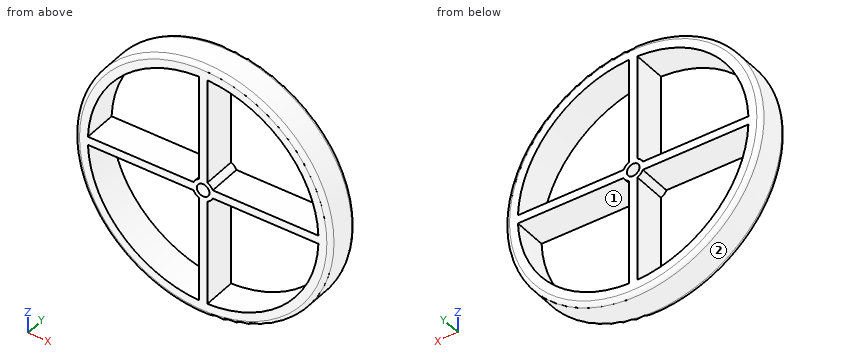
```python
from build123d import *

# Parameters (mm, degrees)
F0_R     = 30.5
F0_R_2   = 1.5000000096
F1_DEPTH = 4
F2_R     = 1


with BuildPart() as f1:
    # F0 (on Front) → F1 (new body, symmetric)
    with BuildSketch(Plane.XZ):
        Circle(F0_R)
        with BuildLine():
            Line((-27.4818121673, -1), (-2.2912878475, -1))
            ThreePointArc((-2.2912878475, -1), (-1.767766953, -1.767766953), (-1, -2.2912878475))
            Line((-1, -2.2912878475), (-1, -27.4818121673))
            ThreePointArc((-1, -27.4818121673), (-19.4454364826, -19.4454364826), (-27.4818121673, -1))
        make_face(mode=Mode.SUBTRACT)
        with BuildLine():
            ThreePointArc((1, -2.2912878475), (1.767766953, -1.767766953), (2.2912878475, -1))
            Line((2.2912878475, -1), (27.4818121673, -1))
            ThreePointArc((27.4818121673, -1), (19.4454364826, -19.4454364826), (1, -27.4818121673))
            Line((1, -27.4818121673), (1, -2.2912878475))
        make_face(mode=Mode.SUBTRACT)
        with BuildLine():
            ThreePointArc((-1, 2.2912878475), (-1.767766953, 1.767766953), (-2.2912878475, 1))
            Line((-2.2912878475, 1), (-27.4818121673, 1))
            ThreePointArc((-27.4818121673, 1), (-19.4454364826, 19.4454364826), (-1, 27.4818121673))
            Line((-1, 27.4818121673), (-1, 2.2912878475))
        make_face(mode=Mode.SUBTRACT)
        Circle(F0_R_2, mode=Mode.SUBTRACT)
        with BuildLine():
            ThreePointArc((1, 27.4818121673), (19.4454364826, 19.4454364826), (27.4818121673, 1))
            Line((27.4818121673, 1), (2.2912878475, 1))
            ThreePointArc((2.2912878475, 1), (1.767766953, 1.767766953), (1, 2.2912878475))
            Line((1, 2.2912878475), (1, 27.4818121673))
        make_face(mode=Mode.SUBTRACT)
    extrude(amount=F1_DEPTH, both=True)

    # F2
    f2_edges = [f1.edges().sort_by_distance(p)[0] for p in [
        (-30.5, -4, 0),
        (-30.5, 4, 0),
    ]]
    fillet(f2_edges, radius=F2_R)


solid = f1.part
```
Here's how the part is built. I have some questions about the finished solid (model axes, mm). Face numbers are marked on the shaded views. Give positions to 0.01 mm unless a question says otherwise; leave off trailing zeros. Write each loop counter-clockwise with the first axis right and the second up, starting at its lowest first coordinate (ties: lowest second). Pieces come first, ordered by that corner, then holes. Notation, with made-up numbers: (59.25, 89) -> (108.25, 89) arc R30 ccw to (108.25, 119) -> close; hole circle Ø11 at (1.25, 4.5). An arc over 180 degrees is marked (long way). Use one line per item in the form item = value.
1) Suppose I cut it at C-C (y = 1.5). Please give me the cut outline in (x, z), and give its area (3 significant figures).
Verdict:
outline = circle Ø61 at (0, 0); hole (-27.48, -1) arc R27.5 ccw to (-1, -27.48) -> (-1, -2.29) arc R2.5 cw to (-2.29, -1) -> close; hole (-27.48, 1) -> (-2.29, 1) arc R2.5 cw to (-1, 2.29) -> (-1, 27.48) arc R27.5 ccw to start; hole circle Ø3 at (0, 0); hole (1, -27.48) arc R27.5 ccw to (27.48, -1) -> (2.29, -1) arc R2.5 cw to (1, -2.29) -> close; hole (1, 2.29) arc R2.5 cw to (2.29, 1) -> (27.48, 1) arc R27.5 ccw to (1, 27.48) -> close
area = 760 mm2
2) Suppose I cut it at A-A (x = 0). Please give me the cut outline in (y, z).
Verdict:
outline = (-4, -29.5) arc R1 ccw to (-3, -30.5) -> (3, -30.5) arc R1 ccw to (4, -29.5) -> (4, -1.5) -> (-4, -1.5) -> close; (-4, 1.5) -> (4, 1.5) -> (4, 29.5) arc R1 ccw to (3, 30.5) -> (-3, 30.5) arc R1 ccw to (-4, 29.5) -> close
3) We'd pull the mould along X, two halves only. Please class the marked faces 1 and 2: +X half, -X half, draft (parallel to the pull), parting line (faces both ways), or undercut.
Verdict:
face_1 = undercut
face_2 = parting line
4) I'm going to push flat-ended pins straight in: pin 1 (1.5 mm diameter, centred on x = -11, y = -2.5, fed in from -Z); pin 2 (2.5 mm diameter, centred on y = -1.5, z = -8.5, fed in from +X); pin 3 (4 mm diameter, centred on y = 1, z = 14.5, fed in from +X). Where does each tip first touch, or does it pass through?
Verdict:
pin_1 = -28.73
pin_2 = 29.63
pin_3 = 27.82
5) If I drill on L1, parallel to Z at x = 0, y = 2.75; L2, parallel to X at y = 3.75, z = -3.5; L3, parallel to Z at x = 17, y = 3, over which ranges is the centre line in solid material (lowest first)? Write a range as [from, to].
Verdict:
L1 = [-30.5, -1.5], [1.5, 30.5]
L2 = [-29.96, -27.28], [-1, 1], [27.28, 29.96]
L3 = [-25.32, -21.62], [-1, 1], [21.62, 25.32]
6) Suppose I cut it at D-D (z = -23). Give the number of separate pieces and of enclosed holes in the cut face, and give its area (3 significant figures).
Verdict:
separate_pieces = 3
enclosed_holes = 0
area = 94.0 mm2
7) Suppose I cut it at B-B (z = 0). Please give me the cut outline in (x, y).
Verdict:
outline = (-30.5, -3) arc R1 ccw to (-29.5, -4) -> (-1.5, -4) -> (-1.5, 4) -> (-29.5, 4) arc R1 ccw to (-30.5, 3) -> close; (1.5, -4) -> (29.5, -4) arc R1 ccw to (30.5, -3) -> (30.5, 3) arc R1 ccw to (29.5, 4) -> (1.5, 4) -> close
